```python
from build123d import *

# Parameters (mm, degrees)
SKETCH_1_W          = 15
SKETCH_1_H          = 30
EXTRUDE_1_DEPTH     = 15
SKETCH_2_R          = 1.1
SKETCH_2_R_2        = 2.1
CUT_EXTRUDE_1_DEPTH = 15
FILLET_2_R          = 25
CUT_EXTRUDE_2_REACH = 117


with BuildPart() as part:
    # 草图1 → 凸台-拉伸1 (new body)
    with BuildSketch(Plane(origin=(0, 0, 0), x_dir=(1, 0, 0), z_dir=(0, 1, 0))):
        with BuildLine():
            Line((55, 0), (0, 0))
            Line((0, 0), (0, -20))
            ThreePointArc((0, -20), (19.968938053, -8.839079645), (42, -15))
            Line((42, -15), (47, -15))
            ThreePointArc((47, -15), (54.5, -10.974937186), (62, -15))
            Line((62, -15), (67, -15))
            ThreePointArc((67, -15), (71, -13), (75, -15))
            Line((75, -15), (110, -15))
            add(Edge.make_bspline(
                [(55, 0), (105, -5), (110, -15)],
                knots=[0, 0, 0, 1, 1, 1], degree=2))
        make_face()
        with Locations((-7.5, -15)):
            Rectangle(SKETCH_1_W, SKETCH_1_H)
    extrude(amount=EXTRUDE_1_DEPTH)

    # 草图2 → 切除-拉伸1 (cut)
    with BuildSketch(Plane(origin=(0, 15, 0), x_dir=(1, 0, 0), z_dir=(0, 1, 0))):
        with Locations(Location((5, -3, 0), (0, 0, 270))):
            Circle(SKETCH_2_R)
        with Locations(Location((10, -3, 0), (0, 0, 270))):
            Circle(SKETCH_2_R)
        with Locations(Location((15, -3, 0), (0, 0, 270))):
            Circle(SKETCH_2_R)
        with Locations(Location((20, -3, 0), (0, 0, 270))):
            Circle(SKETCH_2_R)
        with Locations(Location((25, -3, 0), (0, 0, 270))):
            Circle(SKETCH_2_R)
        with Locations(Location((30, -3, 0), (0, 0, 270))):
            Circle(SKETCH_2_R)
        with Locations(Location((35, -3, 0), (0, 0, 270))):
            Circle(SKETCH_2_R)
        with Locations(Location((40, -3, 0), (0, 0, 270))):
            Circle(SKETCH_2_R)
        with Locations(Location((45, -3, 0), (0, 0, 270))):
            Circle(SKETCH_2_R)
        with Locations(Location((50, -3, 0), (0, 0, 270))):
            Circle(SKETCH_2_R)
        with Locations(Location((55, -3, 0), (0, 0, 270))):
            Circle(SKETCH_2_R)
        with Locations(Location((60, -3, 0), (0, 0, 270))):
            Circle(SKETCH_2_R)
        with Locations(Location((5, -8, 0), (0, 0, 270))):
            Circle(SKETCH_2_R)
        with Locations(Location((10, -8, 0), (0, 0, 270))):
            Circle(SKETCH_2_R)
        with Locations(Location((45, -8, 0), (0, 0, 270))):
            Circle(SKETCH_2_R)
        with Locations(Location((50, -8, 0), (0, 0, 270))):
            Circle(SKETCH_2_R)
        with Locations(Location((55, -8, 0), (0, 0, 270))):
            Circle(SKETCH_2_R)
        with Locations(Location((60, -8, 0), (0, 0, 270))):
            Circle(SKETCH_2_R)
        with Locations(Location((65, -3, 0), (0, 0, 270))):
            Circle(SKETCH_2_R)
        with Locations(Location((65, -8, 0), (0, 0, 270))):
            Circle(SKETCH_2_R)
        with Locations(Location((70, -8, 0), (0, 0, 270))):
            Circle(SKETCH_2_R)
        with Locations(Location((75, -8, 0), (0, 0, 270))):
            Circle(SKETCH_2_R)
        with Locations(Location((-10, -25, 0), (0, 0, 270))):
            Circle(SKETCH_2_R_2)
        with Locations(Location((-10, -17, 0), (0, 0, 270))):
            Circle(SKETCH_2_R_2)
        with Locations(Location((40, -8, 0), (0, 0, 270))):
            Circle(SKETCH_2_R)
        Polygon((88, -12), (85, -8), (88.75, -9), (91, -12), align=None)
        Polygon((94, -12), (92.5, -10), (95, -10.666666667), (96, -12), align=None)
    extrude(amount=-CUT_EXTRUDE_1_DEPTH, mode=Mode.SUBTRACT)

    # 圆角2
    fillet_2_edges = [part.edges().sort_by_distance(p)[0] for p in [
        (-15, 7.5, 0),
    ]]
    fillet(fillet_2_edges, radius=FILLET_2_R)

    # 草图4 → 切除-拉伸2 (cut, up to next)
    with BuildSketch(Plane(origin=(0, 15, 0), x_dir=(1, 0, 0), z_dir=(0, 1, 0)), mode=Mode.PRIVATE) as cut_extrude_2_sk1:
        Polygon((75, -15), (107.538963766, -12.153209548), (110, -12.153209548), (110, -15), align=None)
    cut_extrude_2_tool1 = extrude(cut_extrude_2_sk1.sketch, amount=-CUT_EXTRUDE_2_REACH, mode=Mode.PRIVATE) & part.part
    add(cut_extrude_2_tool1.solids().sort_by_distance((98.27944, 15, 13.988729))[0], mode=Mode.SUBTRACT)


solid = part.part
```
The model under review builds one solid part; all positions refer to its coordinate system, in mm. A direction names the side the tool comes from. Give positions to 0.01 mm unless a question says otherwise; leave off trailing zeros. Write each loop counter-clockwise with the first axis right and the second up, starting at its lowest first coordinate (ties: lowest second). Pieces come first, ordered by that corner, then holes. Notation, with made-up numbers: M 82,27 L 141,27 A17 ccw 141,50 Z; hole C -35.75,66.5 d7. An arc over 180 degrees is marked long. Answer in a Markdown table with one row per item.
Item 1: Add section C-C on y = 6.5. State how many separate pieces and enclosed holes the cut face has, plus the area to 3 significant figures.
Check sheet entries:
| item | result |
|---|---|
| separate pieces | 1 |
| enclosed holes | 27 |
| area | 1,330 mm2 |
Item 2: Add section B-B on z = 17. Give the boundary of the cut face in (x, y).
Check sheet entries:
| item | result |
|---|---|
| outline | M -13.69,0 L -12.1,0 L -12.1,15 L -13.69,15 Z; M -7.9,0 L 2.73,0 L 2.73,15 L -7.9,15 Z |
Item 3: Add section D-D on x = 50. Give the boundary of the cut face in (y, z), plus the area to 3 significant figures.
Check sheet entries:
| item | result |
|---|---|
| outline | M 0,0 L 15,0 L 15,1.9 L 0,1.9 Z; M 0,4.1 L 15,4.1 L 15,6.9 L 0,6.9 Z; M 0,9.1 L 15,9.1 L 15,12.18 L 0,12.18 Z |
| area | 117 mm2 |
Item 4: Tool access review of faces 4 (the face through (44, 7, 15)), 5 (the face through (-9.369, 7.605, 27.003)): name each direction out of +Z, -Z, +X, -X, +Y, -Y from which nothing blocks a thin tool from reaching the whole face with its end or side.
Check sheet entries:
| item | result |
|---|---|
| face 4 | +Z, +X, +Y, -Y |
| face 5 | +Y, -Y |
Item 5: For P1, Ø2, axis at y = 7, z = 14.5, coming from the -X side; P2, Ø2, axis at x = 95, y = 8, coming from the -Z side; P3, Ø4, axis at x = 64.5, y = 9.5, coming from the +Z side, all flat-tipped, find the tip position at first contact; note any pin that passes through.
Check sheet entries:
| item | result |
|---|---|
| P1 | x = -13.12 |
| P2 | z = 6.32 |
| P3 | z = 15 |
Item 6: For line 1 along Z through (x, y) = (65.5, 5.25); line 2 along Z through (x, y) = (90, 11.25); line 3 along X through (y, z) = (6.75, 23.5), list the stretches that pass through material, from the lowest coordinate up.
Check sheet entries:
| item | result |
|---|---|
| line 1 | 1.17 to 2.02, 3.98 to 7.02, 8.98 to 15 |
| line 2 | 5.3 to 10.67, 12 to 13.69 |
| line 3 | -14.95 to -11.47, -8.53 to 0 |
Item 7: Draft analysis for pull direction Z (two halves, no side actions). For faces 1 (the face through (54.376, 7.395, 10.976)), 2 (the face through (-7.482, 7.605, 7.129)), 3 (the face through (40.93, 7.6, 3.59)), state which applies: +Z half, -Z half, draft (parallel to the pull), parting line (faces both ways), or undercut.
Check sheet entries:
| item | result |
|---|---|
| face 1 | +Z half |
| face 2 | -Z half |
| face 3 | undercut |
Item 8: Add section A-A on x = 25. Give the boundary of the cut face in (y, z).
Check sheet entries:
| item | result |
|---|---|
| outline | M 0,0 L 15,0 L 15,1.9 L 0,1.9 Z; M 0,4.1 L 15,4.1 L 15,8.67 L 0,8.67 Z |
